Here's how the part is built. I have some questions about the finished solid (model axes, mm). Face numbers are marked on the shaded views. A direction names the side the tool comes from. Coordinates: 2 decimals unless noted, no trailing zeros. Write each loop counter-clockwise with the first axis right and the second up, starting at its lowest first coordinate (ties: lowest second). Pieces come first, ordered by that corner, then holes.
Item 1: If we section it at B-B (x = -14.5): Please give me the cut outline in (y, z) (1 decimal).
Item 2: For the marked faces 4 and 5, which set-ups out of +Z, -Z, +X, -X, +Y, -Y let a thin tool reach every point of the face, with its end or its side?
Item 3: If we section it at A-A (z = -20): Please give me the cut outline in (x, y) (3 decimals).
Item 4: We'd pull the mould along Z, two halves only. Please class the marked faces 1, 2 and 3: +Z half, -Z half, draft (parallel to the pull), parting line (faces both ways), or undercut.
Item 5: If I drill on line 1 (Y direction, x = -15.5, z = 15) (3 decimals); line 2 (X direction, y = -23, z = -5); line 3 (X direction, y = -20, z = 17.5), over which ranges is the centre line in solid material (lowest first)?
Item 6: I'm going to push flat-ended pins straight in: pin 1 Ø12 at (x, z) = (1, -7) entering from -Y (3 decimals); pin 2 Ø12 at (y, z) = (-17.5, 5) entering from +X (3 decimals); pin 3 Ø8 at (x, y) = (-17, -16) entering from -Z. Where does each tip first touch, or does it pass through?
Item 7: If we section it at C-C (y = -5.25): Please give me the cut outline in (x, z) (3 decimals).
from build123d import *

# Parameters (mm, degrees)
F0_R     = 25.4
F0_R_2   = 20.955
F0_R_3   = 19.05
F0_R_4   = 0.79375
F0_R_5   = 1.27
F1_DEPTH = 3.175
F2_DEPTH = 25.4
F3_R     = 2.038323
F4_DEPTH = 25.4


with BuildPart() as f1:
    # F0 (on Front) → F1 (new body)
    with BuildSketch(Plane.XZ):
        Circle(F0_R)
        Circle(F0_R_2, mode=Mode.SUBTRACT)
        Circle(F0_R_3)
        with Locations((-4.627904, -6.448753)):
            Circle(F0_R_4, mode=Mode.SUBTRACT)
        with Locations((-7.832379, -1.287535)):
            Circle(F0_R_4, mode=Mode.SUBTRACT)
        Circle(F0_R_5, mode=Mode.SUBTRACT)
        with Locations((1.287535, -7.832379)):
            Circle(F0_R_4, mode=Mode.SUBTRACT)
        with Locations((6.448753, -4.627904)):
            Circle(F0_R_4, mode=Mode.SUBTRACT)
        with Locations((-6.448753, 4.627904)):
            Circle(F0_R_4, mode=Mode.SUBTRACT)
        with Locations((-1.287535, 7.832379)):
            Circle(F0_R_4, mode=Mode.SUBTRACT)
        with Locations((7.832379, 1.287535)):
            Circle(F0_R_4, mode=Mode.SUBTRACT)
        with Locations((4.627904, 6.448753)):
            Circle(F0_R_4, mode=Mode.SUBTRACT)
    extrude(amount=F1_DEPTH)

    # F0 (on Front) → F2 (join)
    with BuildSketch(Plane.XZ):
        Circle(F0_R_2)
        Circle(F0_R_3, mode=Mode.SUBTRACT)
    extrude(amount=F2_DEPTH)

    # F3 (on Right) → F4 (cut)
    with BuildSketch(Plane.YZ):
        with Locations((-18.186759, 5.693154)):
            Circle(F3_R)
    extrude(amount=-F4_DEPTH, mode=Mode.SUBTRACT)


solid = f1.part
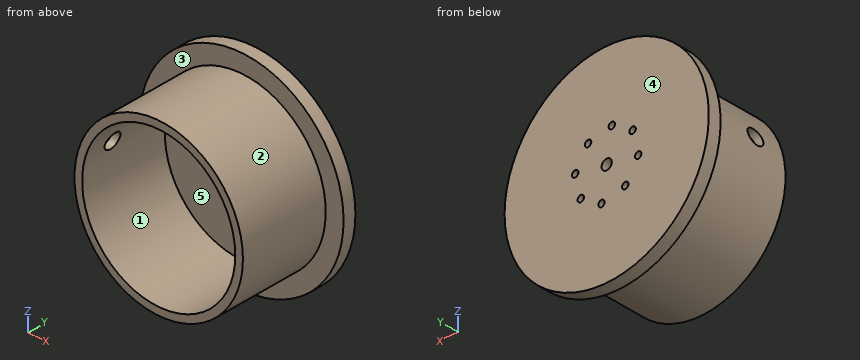
Answer list:
1. outline: (-25.4, -15.1) - (-3.2, -15.1) - (-3.2, -20.9) - (0, -20.9) - (0, 20.9) - (-3.2, 20.9) - (-3.2, 15.1) - (-25.4, 15.1) - (-25.4, 12.4) - (-3.2, 12.4) - (-3.2, -12.4) - (-25.4, -12.4) - close
2. face 4: +Z, -Z, +X, -X, +Y
2. face 5: -Y
3. outline: (-15.658, -3.175) - (-6.254, -3.175) - (-6.254, -25.4) - (6.254, -25.4) - (6.254, -3.175) - (15.658, -3.175) - (15.658, 0) - (-15.658, 0) - close
4. face 1: undercut
4. face 2: parting line
4. face 3: draft
5. line 1: y = -3.175 to 0
5. line 2: x = -20.35 to -18.38, 18.38 to 20.35
5. line 3: x = -11.53 to -7.53, 7.53 to 11.53
6. pin 1: stops at y = -3.175
6. pin 2: stops at x = 20.955
6. pin 3: stops at z = -16.44
7. outline: circle Ø41.91 at (0, 0); hole circle Ø38.1 at (0, 0)
